from build123d import *

# Parameters (mm, degrees)
SKETCH2_W           = 100
SKETCH2_H           = 125
SKETCH2_R           = 1.5
SKETCH2_R_2         = 2.5
BOSS_EXTRUDE1_DEPTH = 8
SKETCH5_W           = 100
SKETCH5_H           = 10
BOSS_EXTRUDE2_DEPTH = 35
SKETCH7_R           = 10
SKETCH7_R_2         = 3.75
CUT_EXTRUDE2_DEPTH  = 290
SKETCH8_R           = 18.5
CUT_EXTRUDE5_DEPTH  = 133.566964211
SKETCH9_R           = 2.5
CUT_EXTRUDE6_DEPTH  = 20


with BuildPart() as part:
    # Sketch2 → Boss-Extrude1 (new body)
    with BuildSketch(Plane.XY):
        with Locations((0, 17.5)):
            Rectangle(SKETCH2_W, SKETCH2_H)
        with Locations(Location((-9, -8.03563588, 0), (0, 0, 180))):
            Circle(SKETCH2_R, mode=Mode.SUBTRACT)
        with Locations(Location((9, -31.96436412, 0), (0, 0, 180))):
            Circle(SKETCH2_R, mode=Mode.SUBTRACT)
        with Locations((9, -8.03563588)):
            Circle(SKETCH2_R, mode=Mode.SUBTRACT)
        with Locations((-9, -31.96436412)):
            Circle(SKETCH2_R, mode=Mode.SUBTRACT)
        with Locations(Location((9, 43.03563588, 0), (0, 0, 180))):
            Circle(SKETCH2_R, mode=Mode.SUBTRACT)
        with Locations((-9, 43.03563588)):
            Circle(SKETCH2_R, mode=Mode.SUBTRACT)
        with Locations(Location((-9, 66.96436412, 0), (0, 0, 180))):
            Circle(SKETCH2_R, mode=Mode.SUBTRACT)
        with Locations((9, 66.96436412)):
            Circle(SKETCH2_R, mode=Mode.SUBTRACT)
        with Locations((0, 33.18)):
            Circle(SKETCH2_R_2, mode=Mode.SUBTRACT)
        with Locations((0, 1.82)):
            Circle(SKETCH2_R_2, mode=Mode.SUBTRACT)
    extrude(amount=BOSS_EXTRUDE1_DEPTH)

    # Sketch5 → Boss-Extrude2 (add)
    with BuildSketch(Plane.XY.offset(8)):
        with Locations((0, 75)):
            Rectangle(SKETCH5_W, SKETCH5_H)
        with Locations((0, -40)):
            Rectangle(SKETCH5_W, SKETCH5_H)
    extrude(amount=BOSS_EXTRUDE2_DEPTH)

    # Sketch7 → Cut-Extrude2 (cut)
    with BuildSketch(Plane(origin=(0, 80, 0), x_dir=(1, 0, 0), z_dir=(0, 1, 0))):
        with Locations(Location((-3.365, -21.5, 0), (0, 0, 270))):
            Circle(SKETCH7_R)
        with Locations(Location((-40.365, -21.5, 0), (0, 0, 270))):
            Circle(SKETCH7_R_2)
        with Locations(Location((33.635, -21.5, 0), (0, 0, 270))):
            Circle(SKETCH7_R_2)
    extrude(amount=-CUT_EXTRUDE2_DEPTH, mode=Mode.SUBTRACT)

    # Sketch8 → Cut-Extrude5 (cut, through all)
    with BuildSketch(Plane(origin=(0, -35, 0), x_dir=(1, 0, 0), z_dir=(0, 1, 0))):
        with Locations((-3.365, -51.164787316)):
            Circle(SKETCH8_R)
    extrude(amount=-CUT_EXTRUDE5_DEPTH, mode=Mode.SUBTRACT)

    # Sketch9 → Cut-Extrude6 (cut)
    with BuildSketch(Plane(origin=(0, 80, 0), x_dir=(1, 0, 0), z_dir=(0, 1, 0))):
        with Locations(Location((-3.365, -5.73, 0), (0, 0, 270))):
            Circle(SKETCH9_R)
        with Locations(Location((12.405, -21.5, 0), (0, 0, 270))):
            Circle(SKETCH9_R)
        with Locations(Location((-19.135, -21.5, 0), (0, 0, 180))):
            Circle(SKETCH9_R)
        with Locations(Location((-3.365, -37.27, 0), (0, 0, 180))):
            Circle(SKETCH9_R)
    extrude(amount=-CUT_EXTRUDE6_DEPTH, mode=Mode.SUBTRACT)


solid = part.part
Input: part model. Units: mm. Frame: model coordinates. A direction names the side the tool comes from. Coordinates: 2 decimals unless noted, no trailing zeros. Order: outer loops, then holes, each group sorted by start corner. A loop starts at its lowest first (then second) coordinate and runs counter-clockwise, first axis right, second up.
1. Access query for faces 1 (the cylindrical face through (-3.255, 70.14, 3.232)), 2 (the flat face through (10, -35, 25)), 3 (the cylindrical face through (-37.203, -39.93, 23.516)). Directions: +Z, -Z, +X, -X, +Y, -Y. A direction counts if a zero-diameter tool reaches every point of the face in a straight line with its end or side. Return the directions, or none.
Checked values:
face 1: +Y
face 2: +Z, +X, -X
face 3: +Y, -Y
2. Contact query for flat-ended pins moving along their axis: P1, Ø3, axis at x = 0, y = 1.82, coming from the -Z side; P2, Ø3.5, axis at x = 9, y = 66.96, coming from the +Z side. Output: stop coordinate, or through.
Checked values:
P1: passes through
P2: stops at z = 8
3. Cut plane A-A, the plane x = -23.5. Return loops of the section in (y, z), plus the area to 3 significant figures.
Checked values:
outline: (-45, 0) - (80, 0) - (80, 43) - (70, 43) - (70, 8) - (-35, 8) - (-35, 43) - (-45, 43) - close
area: 1,700 mm2
4. Cut plane B-B, the plane z = 37.27. Return loops of the section in (x, y) (3 decimals).
Checked values:
outline: (-50, -45) - (-15.579, -45) - (-15.579, -35) - (-50, -35) - close; (-50, 70) - (-5.865, 70) - (-5.865, 80) - (-50, 80) - close; (-0.865, 70) - (50, 70) - (50, 80) - (-0.865, 80) - close; (8.849, -45) - (50, -45) - (50, -35) - (8.849, -35) - close
5. Cut plane C-C, the plane y = 33.18. Return loops of the section in (x, z), plus the area to 3 significant figures.
Checked values:
outline: (-50, 0) - (-2.5, 0) - (-2.5, 8) - (-50, 8) - close; (2.5, 0) - (50, 0) - (50, 8) - (2.5, 8) - close
area: 760 mm2
6. Draft query along Y for faces 4 (the flat face through (-35, -40, 43)), 5 (the flat face through (-1, 18, 8)), 6 (the flat face through (-3, 60, 6)), 7 (the cylindrical face through (9.33, -30.5, 3.94)). Return one class per face: +Y half, -Y half, draft (parallel to the pull), parting line (faces both ways), or undercut.
Checked values:
face 4: draft
face 5: undercut
face 6: +Y half
face 7: undercut
7. Ray query, line 1 along Y through (x, z) = (30, 8.5); line 2 along Y through (x, z) = (0, 6.75); line 3 along X through (y, z) = (33, 6). Return the intervals inside material, ascending.
Checked values:
line 1: y = -45 to -35, 70 to 80
line 2: y = -45 to -0.68, 4.32 to 30.68, 35.68 to 80
line 3: x = -50 to -2.49, 2.49 to 50
8. Cut plane D-D, the plane x = -9. Count the separate pieces of the cut face and the enclosed holes in it, plus the area to 3 significant figures.
Checked values:
separate pieces: 7
enclosed holes: 0
area: 1,180 mm2
